from build123d import *

# Parameters (mm, degrees)
BOSS_EXTRUDE1_DEPTH = 3.81
BOSS_EXTRUDE2_DEPTH = 3.81


with BuildPart() as part:
    # Sketch2 → Boss-Extrude1 (new body)
    with BuildSketch(Plane(origin=(0, 0, 0), x_dir=(0, 0, -1), z_dir=(1, 0, 0))):
        Polygon((0, 0), (73.406, 0), (73.406, -76.2), (49.276, -76.2), (49.276, -26.924), (0, -26.924), align=None)
    extrude(amount=BOSS_EXTRUDE1_DEPTH)

    # Sketch5 → Boss-Extrude2 (add)
    with BuildSketch(Plane(origin=(0, 0, 0), x_dir=(1, 0, 0), z_dir=(0, 1, 0))):
        Polygon((-69.596, 73.406), (3.81, 73.406), (3.81, 0), (-20.32, 0), (-20.32, 49.276), (-69.596, 49.276), align=None)
    extrude(amount=BOSS_EXTRUDE2_DEPTH)


solid = part.part
Model file for the job. Use its own axes, mm. A direction names the side the tool comes from. Give positions to 0.01 mm unless a question says otherwise; leave off trailing zeros. Loops run counter-clockwise (first coordinate to the right, second up) from the corner with the lowest first, then second, coordinate; pieces in that order, holes last. Notation, with made-up numbers: (11.5, -13.75) -> (68.5, -13.75) arc R24 ccw to (68.5, 18.25) -> close; hole circle Ø6 at (55.5, 75). An arc over 180 degrees is marked (long way). Use a Markdown table: item, result. Add a question column.
(1) Wall check: line 1 along Y through (x, z) = (-16, -43). Give the ranges that are in metal, low to high.
(2) Slice it at B-B on y = -39. List the corners of the cut face in (x, z), and give its area (3 significant figures).
(3) Slice it at A-A on z = -24. List the corners of the cut face in (x, y).
(4) Drop flat-ended pins along their axis: pin 1 Ø1.1 at (x, y) = (1, -51) entering from +Z; pin 2 Ø1.1 at (y, z) = (2, -21) entering from -X; pin 3 Ø12 at (x, z) = (-15, -36.5) entering from -Y. Give the stop position or say it passes through.
(5) Slice it at D-D on z = -60. List the corners of the cut face in (x, y), and give its area (3 significant figures).
(6) Tool access for faces 1 (the flat face through (-19, 0, -45)), 2 (the flat face through (2, -26.924, -25)), 3 (the flat face through (2, -76.2, -62)), 4 (the flat face through (-45, 2, -49.276)): list every direction of +Z, -Z, +X, -X, +Y, -Y with a clear straight run to the whole face (end or side of a thin tool).
Filled sheet:
| question | item | result |
|---|---|---|
| 1 | line 1 | 0 to 3.81 |
| 2 | outline | (0, -73.41) -> (3.81, -73.41) -> (3.81, -49.28) -> (0, -49.28) -> close |
| 2 | area | 91.9 mm2 |
| 3 | outline | (-20.32, 0) -> (0, 0) -> (0, -26.92) -> (3.81, -26.92) -> (3.81, 3.81) -> (-20.32, 3.81) -> close |
| 4 | pin 1 | z = -49.28 |
| 4 | pin 2 | x = -20.32 |
| 4 | pin 3 | y = 0 |
| 5 | outline | (-69.6, 0) -> (0, 0) -> (0, -76.2) -> (3.81, -76.2) -> (3.81, 3.81) -> (-69.6, 3.81) -> close |
| 5 | area | 570 mm2 |
| 6 | face 1 | +Z, -Z, -X, -Y |
| 6 | face 2 | +Z, +X, -X, -Y |
| 6 | face 3 | +Z, -Z, +X, -X, -Y |
| 6 | face 4 | +Z, -X, +Y, -Y |
